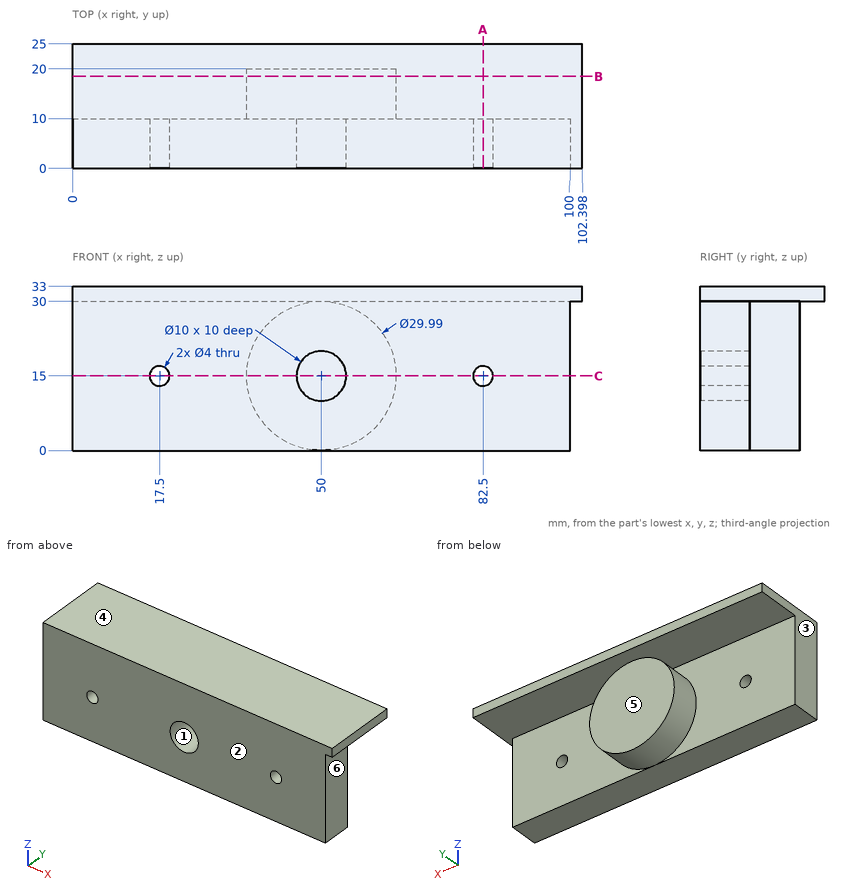
The figure shows three views and two pictorial views of one solid part (mm, origin at its lowest corner). Answer the questions. A direction names the side the tool comes from. Give positions to 0.01 mm unless a question says otherwise; leave off trailing zeros. Write each loop counter-clockwise with the first axis right and the second up, starting at its lowest first coordinate (ties: lowest second). Pieces come first, ordered by that corner, then holes. Notation, with made-up numbers: M -1.5,79 L 33.5,79 A31 ccw 33.5,114 Z; hole C 37.5,-13.5 d9. An arc over 180 degrees is marked long. One line per item, written item: value. Start each with the question number.
(1) A tool of negligible diameter and unlimited length cuts with its end or side. For the marked faces 4, 5 and 6, from which of +Z, -Z, +X, -X, +Y, -Y can it reach the whole face along a straight path? Write none if from no direction.
(2) Flat-ended cylindrical pins translate along their axes: pin 1 Ø1.5 at (x, z) = (81, 3.5) entering from +Y; pin 2 Ø15 at (x, z) = (43, 14.5) entering from +Y; pin 3 Ø12 at (x, y) = (13, 19.5) entering from -Z. Find the tip coordinate at first contact, or state that the pin passes through.
(3) Determine the mould class of the marked faces 1, 2 and 3 for opening direction X: pulls with the +X half, pulls with the -X half, needs draft (parallel to the pull), parting line crosses it, or undercut.
(4) Find the intervals of material crossed by line 1 (Z direction, x = 17.5, y = 3); line 2 (Z direction, x = 50, y = 2); line 3 (Z direction, x = 27, y = 15), in increasing order.
(5) Find section B-B (y = 18.5). Determine the outline of the cut face in (x, z) (1 decimal).
(6) Find section C-C (z = 15). Determine the outline of the cut face in (x, y) (1 decimal), plus the area to 3 significant figures.
(7) Find section A-A (x = 82.5). Determine the outline of the cut face in (y, z), plus the area to 3 significant figures.
Results below:
1. face 4: +Z, +X, -X, +Y, -Y
1. face 5: -Z, +X, -X, +Y
1. face 6: -Z, +X, +Y, -Y
2. pin 1: stops at y = 10
2. pin 2: stops at y = 20
2. pin 3: stops at z = 30
3. face 1: undercut
3. face 2: needs draft
3. face 3: pulls with the -X half
4. line 1: z = 0 to 13, 17 to 33
4. line 2: z = 0 to 10, 20 to 33
4. line 3: z = 30 to 33
5. outline: M 0,30 L 102.4,30 L 102.4,33 L 0,33 Z; C 50,15 d30
6. outline: M 0,0 L 15.5,0 L 15.5,10 L 0,10 Z; M 19.5,0 L 45,0 L 45,10 L 55,10 L 55,0 L 80.5,0 L 80.5,10 L 65,10 L 65,20 L 35,20 L 35,10 L 19.5,10 Z; M 84.5,0 L 100,0 L 100,10 L 84.5,10 Z
6. area: 1,120 mm^2
7. outline: M 0,0 L 10,0 L 10,13 L 0,13 Z; M 0,17 L 10,17 L 10,30 L 25,30 L 25,33 L 0,33 Z
7. area: 335 mm^2
